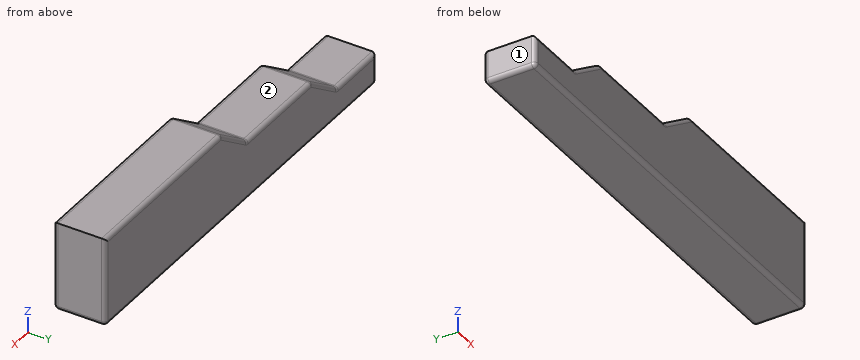
```python
from build123d import *

# Parameters (mm, degrees)
F1_DEPTH = 25
F2_R     = 2


with BuildPart() as f1:
    # F0 (on Front) → F1 (new body)
    with BuildSketch(Plane.XZ):
        Polygon((0, 15), (0, 0), (210, 0), (210, 43.008302), (120, 43.008302), (100, 29.004151), (50, 29.004151), (30, 15), align=None)
    extrude(amount=F1_DEPTH)

    # F2
    f2_edges = [f1.edges().sort_by_distance(p)[0] for p in [
        (165, -25, 43.008302),
        (165, 0, 43.008302),
        (210, -25, 21.504151),
        (210, 0, 21.504151),
        (210, -12.5, 0),
        (105, -25, 0),
        (110, -25, 36.006226),
        (75, -25, 29.004151),
        (40, -25, 22.002075),
        (15, -25, 15),
        (15, 0, 15),
        (30, -12.5, 15),
        (40, 0, 22.002075),
        (50, -12.5, 29.004151),
        (75, 0, 29.004151),
        (110, 0, 36.006226),
        (100, -12.5, 29.004151),
        (120, -12.5, 43.008302),
        (0, 0, 7.5),
        (0, -12.5, 0),
        (0, -25, 7.5),
        (105, 0, 0),
    ]]
    fillet(f2_edges, radius=F2_R)


solid = f1.part
```
Read the model definition and answer for the solid it produces. Units are mm, in the model's axes. Face numbers are marked on the shaded views. A direction names the side the tool comes from. Coordinates: 2 decimals unless noted, no trailing zeros. Loops run counter-clockwise (first coordinate to the right, second up) from the corner with the lowest first, then second, coordinate; pieces in that order, holes last. Notation, with made-up numbers: (71.25, 11.5) -> (76.25, 11.5) arc R19 ccw to (76.25, 43.5) -> close; hole circle Ø6 at (85, -26). An arc over 180 degrees is marked (long way). Return JSON: item names as keys, results as strings.
Item 1: For the marked faces 1 and 2, determine the directions among +Z, -Z, +X, -X, +Y, -Y from which every point of the face is accessible in a straight line to the end or side of a thin tool.
Answers:
{"face 1": "+Z, -Z, -X, +Y, -Y", "face 2": "+Z, -X, +Y, -Y"}
Item 2: Flat-ended cylindrical pins translate along their axes: P1, Ø1, axis at x = 120, y = -11, coming from the +Z side; P2, Ø4, axis at x = 95, y = -5, coming from the +Z side. Find the tip coordinate at first contact, or state that the pin passes through.
Answers:
{"P1": "stops at z = 43", "P2": "stops at z = 29"}
Item 3: Find section A-A (x = 73). Determine the outline of the cut face in (y, z), plus the area to 3 significant figures.
Answers:
{"outline": "(-25, 2) arc R2 ccw to (-23, 0) -> (-2, 0) arc R2 ccw to (0, 2) -> (0, 27) arc R2 ccw to (-2, 29) -> (-23, 29) arc R2 ccw to (-25, 27) -> close", "area": "722 mm2"}
Item 4: Find the intervals of material crossed by probe 1 along Z at (x, y) = (59.5, -4.75); probe 2 along Z at (x, y) = (25, -6.25); probe 3 along X at (y, z) = (-9.25, 39), in increasing order.
Answers:
{"probe 1": "z = 0 to 29", "probe 2": "z = 0 to 15", "probe 3": "x = 114.28 to 210"}
Item 5: Find section B-B (y = -12). Determine the outline of the cut face in (x, z).
Answers:
{"outline": "(0, 2) arc R2 ccw to (2, 0) -> (208, 0) arc R2 ccw to (210, 2) -> (210, 43.01) -> (120.63, 43.01) arc R2 ccw to (119.48, 42.65) -> (100.52, 29.37) arc R2 cw to (99.37, 29) -> (50.63, 29) arc R2 ccw to (49.48, 28.64) -> (30.52, 15.36) arc R2 cw to (29.37, 15) -> (0, 15) -> close"}
